Job drawing, mm, ordinate dimensions from the low corner. One solid piece. Round coordinates to 2 decimals unless told otherwise and drop trailing zeros. Write each loop counter-clockwise with the first axis right and the second up, starting at its lowest first coordinate (ties: lowest second). Pieces come first, ordered by that corner, then holes. Notation, with made-up numbers: (69.5, 33.5) - (95.5, 33.5) arc R19 ccw to (95.5, 53.5) - close; hole circle Ø11 at (-9, 29). An arc over 180 degrees is marked (long way). Write each question's results on one line, items separated by ' | '.
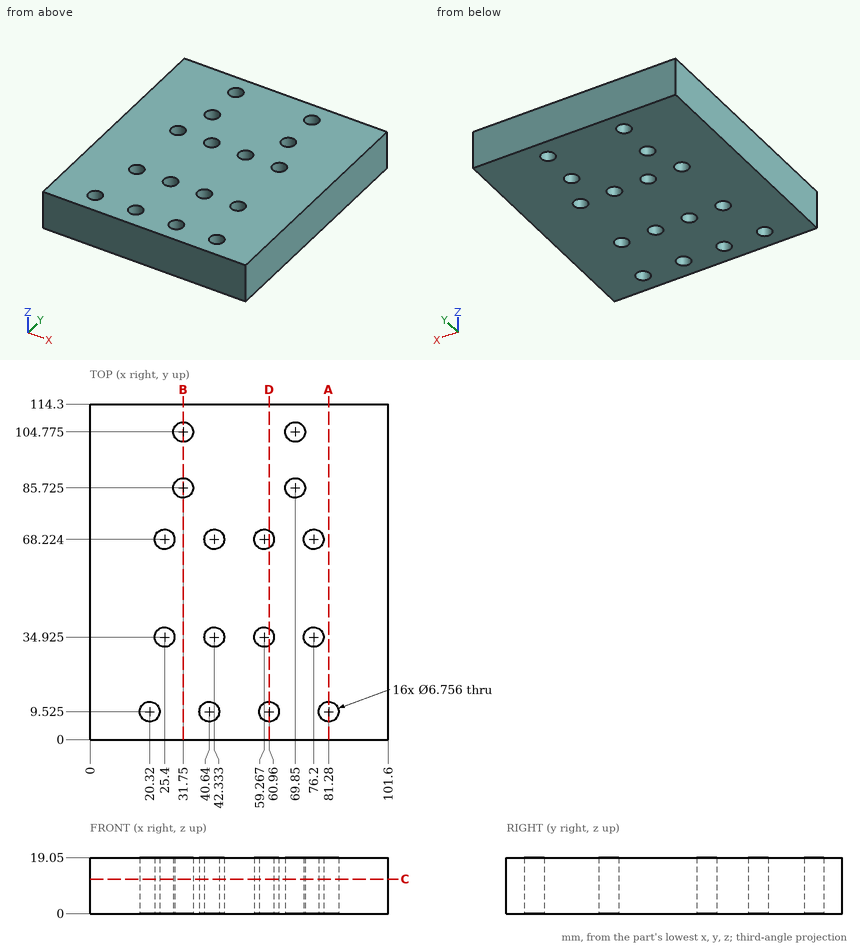
(1) Drill centre lines: probe 1 along Y at (x, z) = (25.4, 11); probe 2 along Y at (x, z) = (69.85, 8); probe 3 along Y at (x, z) = (81.28, 9). Where is each one in solid material? Low to high. Write a range as [from, to].
Worked answers:
probe 1: y = [0, 31.55], [38.3, 64.85], [71.6, 114.3] | probe 2: y = [0, 82.35], [89.1, 101.4], [108.15, 114.3] | probe 3: y = [0, 6.15], [12.9, 114.3]
(2) Slice it at B-B, the plane x = 31.75. Write the cut outline in (y, z), and give its area (3 significant figures).
Worked answers:
outline: (0, 0) - (82.35, 0) - (82.35, 19.05) - (0, 19.05) - close; (89.1, 0) - (101.4, 0) - (101.4, 19.05) - (89.1, 19.05) - close; (108.15, 0) - (114.3, 0) - (114.3, 19.05) - (108.15, 19.05) - close | area: 1,920 mm2
(3) Slice it at A-A, the plane x = 81.28. Write the cut outline in (y, z).
Worked answers:
outline: (0, 0) - (6.15, 0) - (6.15, 19.05) - (0, 19.05) - close; (12.9, 0) - (114.3, 0) - (114.3, 19.05) - (12.9, 19.05) - close
(4) Slice it at D-D, the plane x = 60.96. Write the cut outline in (y, z).
Worked answers:
outline: (0, 0) - (6.15, 0) - (6.15, 19.05) - (0, 19.05) - close; (12.9, 0) - (32, 0) - (32, 19.05) - (12.9, 19.05) - close; (37.85, 0) - (65.3, 0) - (65.3, 19.05) - (37.85, 19.05) - close; (71.15, 0) - (114.3, 0) - (114.3, 19.05) - (71.15, 19.05) - close
(5) Flat gauge pin, fed straight in: pin 1 Ø5.5 at (x, y) = (31.75, 104.775) entering from +Z. Where does the tip first touch, or does it go through?
Worked answers:
pin 1: passes through
(6) Slice it at C-C, the plane z = 11.75. State how many separate pieces and enclosed holes the cut face has, and give its area (3 significant figures).
Worked answers:
separate pieces: 1 | enclosed holes: 16 | area: 11,000 mm2
